Autodesk Fusion 360 part; units mm, degrees
sketch "Sketch1" plane through (0, 0, 0) normal (0, 0, 1) x (1, 0, 0)
  line L0 (0, 0) -> (40, 0)
  line L1 (40, 0) -> (40, 15)
  line L2 (40, 15) -> (0, 15)
  line L3 (0, 15) -> (0, 0)
  dimension "d1" = 40
  dimension "d2" = 15
extrude "Extrude1" add sketch "Sketch1" along normal blind 2.5
sketch "Sketch2" plane through (0, 0, 2.5) normal (0, 0, 1) x (-1, 0, 0)
  line L0 (0, -15) -> (0, 0)
  line L1 (0, 0) -> (-40, 0)
  line L2 (-40, 0) -> (-40, -15)
  line L3 (-40, -15) -> (0, -15)
  line L4 (-20, -20) -> (-20, 7) construction
  line L5 (-32, -20) -> (-32, 13) construction
  line L6 (-8, -20) -> (-8, 12) construction
  line L7 (2.5927, -7.5) -> (-48, -7.5) construction
  line L8 (-13, -8.1) -> (-13, -6.9)
  line L9 (-27, -8.1) -> (-27, -6.9)
  arc A0 (-11.5496, -8.1) -> (-11.5496, -6.9) centre (-8, -7.5) ccw
  line L10 (-28.4504, -6.9) -> (-27, -6.9)
  line L11 (-13, -6.9) -> (-11.5496, -6.9)
  line L12 (-11.5496, -8.1) -> (-13, -8.1)
  line L13 (-27, -8.1) -> (-28.4504, -8.1)
  arc A1 (-28.4504, -6.9) -> (-28.4504, -8.1) centre (-32, -7.5) ccw
  dimension "d5" = 20
  dimension "d6" = 12
  dimension "d7" = 12
  dimension "d8" = 7.5
  dimension "d9" = 7.2
  dimension "d10" = 7.2
  dimension "d12" = 0.6
  dimension "d13" = 5
  dimension "d14" = 5
extrude "Extrude2" cut sketch "Sketch2" against normal blind 4 contours L8 A0 L11 L12 | L9 L10 L13 A1
fillet "Fillet1" radius 5 1 edges at (0, 0, 1.25)
fillet "Fillet2" radius 5 2 edges at (40, 0, 1.25) (40, 15, 1.25)
fillet "Fillet3" radius 5 1 edges at (0, 15, 1.25)
Read the model definition and answer for the solid it produces. Units are mm, in the model's axes. A direction names the side the tool comes from. Give positions to 0.01 mm unless a question says otherwise; leave off trailing zeros. Loops run counter-clockwise (first coordinate to the right, second up) from the corner with the lowest first, then second, coordinate; pieces in that order, holes last. Notation, with made-up numbers: (29.5, 29) - (40.5, 29) arc R30 cw to (40.5, 51) - close; hole circle Ø5 at (-16, 52). An arc over 180 degrees is marked (long way). Answer as CSV lines item,"result". Start each with the question number.
1) Straight lines are drawn through the part: L1, parallel to X at y = 7.5, z = 0.75; L2, parallel to Y at x = 8, z = 1.85; L3, parallel to X at y = 6.25, z = 0.1. For each, find the intervals that lie inside material, in ascending order. Write a range as from..to.
2) Find section B-B (y = 7.5). Write down the section's boundary in (x, z), then the cut area to 3 significant figures.
3) Find section D-D (y = 2). Write down the section's boundary in (x, z), then the cut area to 3 significant figures.
4) Which of the six approach directions +Z, -Z, +X, -X, +Y, -Y give full straight-line access (tool end or side, diameter ignored) to faces 1 (the face through (20, 15, 1)), 2 (the face through (28, 8.1, 1))?
5) Find section A-A (z = 0.8). Write down the section's boundary in (x, y), then the cut area to 3 significant figures.
6) Determine the mould class of faces 3 (the face through (13, 7.5, 1.3)), 4 (the face through (1, 2, 1)), 5 (the face through (20, 8, 2.5)) for opening direction Y: released by +Y, released by -Y, zero draft, split by the parting line, or undercut.
7) Find section C-C (x = 8). Write down the section's boundary in (y, z).
8) This flat-tipped pin is pushed along its axis until it touches: pin 1 Ø4.5 at (x, y) = (32, 7.5) entering from -Z. Where does it stop, or does it pass through?
Findings below:
1,L1,"0..4.4, 13..27, 35.6..40"
1,L2,"0..3.9, 11.1..15"
1,L3,"0..4.62, 11.38..28.62, 35.38..40"
2,outline,"(0, 0) - (4.4, 0) - (4.4, 2.5) - (0, 2.5) - close; (13, 0) - (27, 0) - (27, 2.5) - (13, 2.5) - close; (35.6, 0) - (40, 0) - (40, 2.5) - (35.6, 2.5) - close"
2,area,"57.0 mm^2"
3,outline,"(1, 0) - (39, 0) - (39, 2.5) - (1, 2.5) - close"
3,area,"95.0 mm^2"
4,face 1,"+Z, -Z, +X, -X, +Y"
4,face 2,"+Z, -Z"
5,outline,"(0, 5) arc R5 ccw to (5, 0) - (35, 0) arc R5 ccw to (40, 5) - (40, 10) arc R5 ccw to (35, 15) - (5, 15) arc R5 ccw to (0, 10) - close; hole (11.55, 6.9) - (13, 6.9) - (13, 8.1) - (11.55, 8.1) arc R3.6 ccw (long way) to start; hole (27, 6.9) - (28.45, 6.9) arc R3.6 ccw (long way) to (28.45, 8.1) - (27, 8.1) - close"
5,area,"494 mm^2"
6,face 3,"undercut"
6,face 4,"released by -Y"
6,face 5,"zero draft"
7,outline,"(0, 0) - (3.9, 0) - (3.9, 2.5) - (0, 2.5) - close; (11.1, 0) - (15, 0) - (15, 2.5) - (11.1, 2.5) - close"
8,pin 1,"through"
